from build123d import *

# Parameters (mm, degrees)
SKETCH_1_R        = 2.25
SKETCH_1_R_2      = 1.7
EXTRUDE_237_DEPTH = 6


with BuildPart() as part:
    # 草图1 → Extrude 237 (new body)
    with BuildSketch(Plane.XY):
        Polygon((-22, -17), (-17, -22), (21, -22), (39, -10), (99, -8), (108, -5), (108, 5), (99, 8), (39, 10), (21, 22), (-17, 22), (-22, 17), align=None)
        with Locations((-8.85, -8.85)):
            Circle(SKETCH_1_R, mode=Mode.SUBTRACT)
        with Locations((-8.85, 8.85)):
            Circle(SKETCH_1_R, mode=Mode.SUBTRACT)
        with Locations((8.85, -8.85)):
            Circle(SKETCH_1_R, mode=Mode.SUBTRACT)
        with Locations((8.85, 8.85)):
            Circle(SKETCH_1_R, mode=Mode.SUBTRACT)
        with Locations((100, 0)):
            Circle(SKETCH_1_R_2, mode=Mode.SUBTRACT)
    extrude(amount=EXTRUDE_237_DEPTH)


solid = part.part
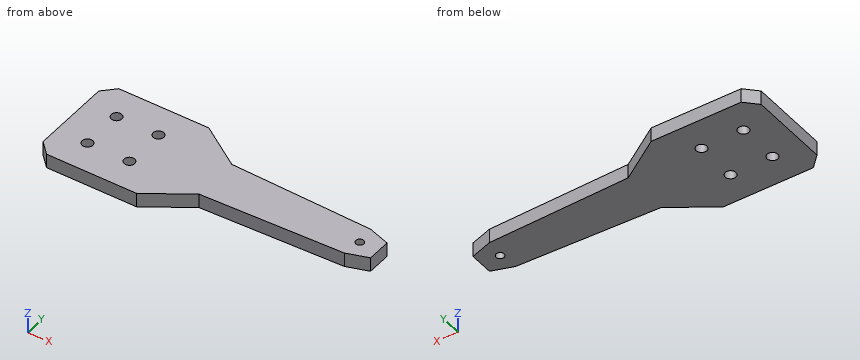
CAD build for the part. Positions are in the model's coordinates, mm. Coordinates: 2 decimals unless noted, no trailing zeros. Order: outer loops, then holes, each group sorted by start corner. A loop starts at its lowest first (then second) coordinate and runs counter-clockwise, first axis right, second up. Notation, with made-up numbers: (-5.5, 31.5) -> (43.5, 31.5) arc R9 cw to (43.5, 40.5) -> close; hole circle Ø9 at (55.25, -20.5). An arc over 180 degrees is marked (long way). Answer in a Markdown table with one row per item.
1) Band-saw the part on A-A (y = 0). List the corners of the cut face in (x, z).
Check values:
| item | result |
|---|---|
| outline | (-22, 0) -> (98.3, 0) -> (98.3, 6) -> (-22, 6) -> close; (101.7, 0) -> (108, 0) -> (108, 6) -> (101.7, 6) -> close |
2) Band-saw the part on D-D (x = 30). List the corners of the cut face in (y, z).
Check values:
| item | result |
|---|---|
| outline | (-16, 0) -> (16, 0) -> (16, 6) -> (-16, 6) -> close |
3) Band-saw the part on B-B (x = -8.85). List the corners of the cut face in (y, z).
Check values:
| item | result |
|---|---|
| outline | (-22, 0) -> (-11.1, 0) -> (-11.1, 6) -> (-22, 6) -> close; (-6.6, 0) -> (6.6, 0) -> (6.6, 6) -> (-6.6, 6) -> close; (11.1, 0) -> (22, 0) -> (22, 6) -> (11.1, 6) -> close |
4) Band-saw the part on C-C (z = 1.5). List the corners of the cut face in (x, y), and give its area (3 significant figures).
Check values:
| item | result |
|---|---|
| outline | (-22, -17) -> (-17, -22) -> (21, -22) -> (39, -10) -> (99, -8) -> (108, -5) -> (108, 5) -> (99, 8) -> (39, 10) -> (21, 22) -> (-17, 22) -> (-22, 17) -> close; hole circle Ø4.5 at (-8.85, -8.85); hole circle Ø4.5 at (-8.85, 8.85); hole circle Ø4.5 at (8.85, -8.85); hole circle Ø4.5 at (8.85, 8.85); hole circle Ø3.4 at (100, 0) |
| area | 3,570 mm2 |
5) Flat gauge pins, fed straight in: P1, Ø3, axis at x = 100, y = 0, coming from the -Z side; P2, Ø1, axis at x = 73.5, z = 5, coming from the -Y side. Where does each tip first touch, or does it go through?
Check values:
| item | result |
|---|---|
| P1 | through |
| P2 | y = -8.87 |
6) Drill centre lines: line 1 (Y direction, x = -8.85, z = 4.4); line 2 (X direction, y = 15, z = 1.95); line 3 (Y direction, x = 58, z = 5.3). Where is each one in solid material? Low to high.
Check values:
| item | result |
|---|---|
| line 1 | -22 to -11.1, -6.6 to 6.6, 11.1 to 22 |
| line 2 | -22 to 31.5 |
| line 3 | -9.37 to 9.37 |
